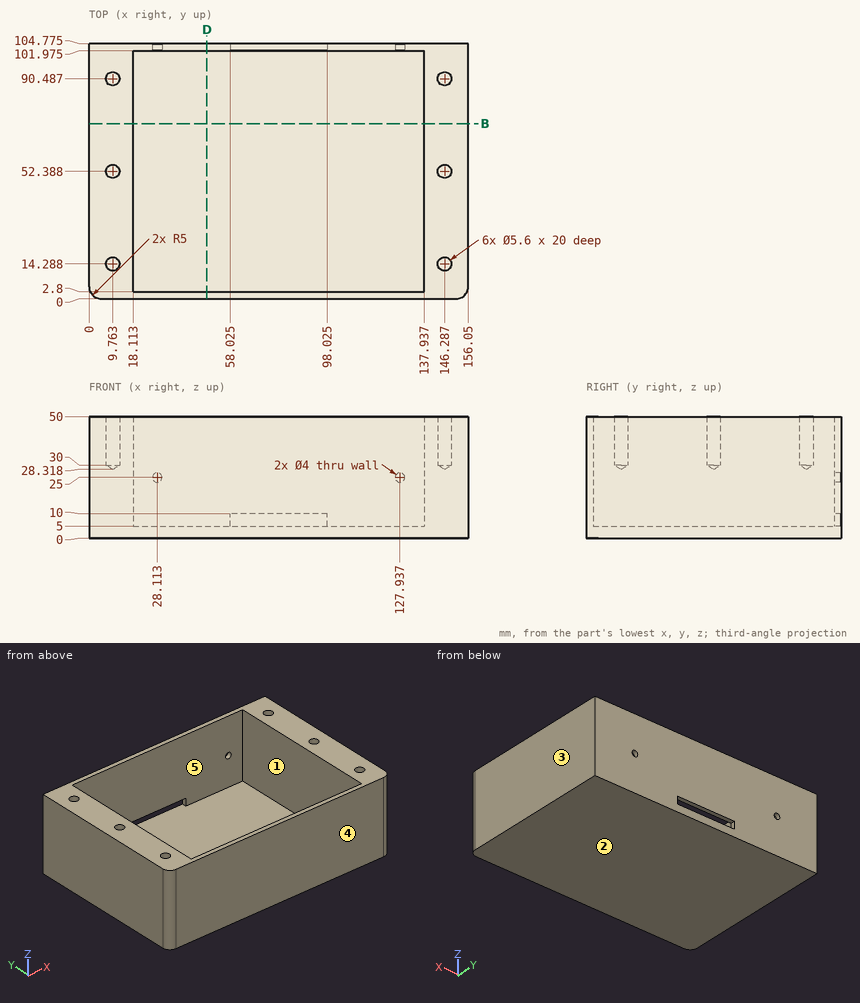
Study the drawing (mm; zero at the part's minimum x, y, z) and answer. A direction names the side the tool comes from. Give positions to 0.01 mm unless a question says otherwise; leave off trailing zeros. Write each loop counter-clockwise with the first axis right and the second up, starting at its lowest first coordinate (ties: lowest second). Pieces come first, ordered by that corner, then holes. Notation, with made-up numbers: (-0.75, -12.5) -> (40.25, -12.5) arc R27 cw to (40.25, 5.5) -> close; hole circle Ø9 at (24, 23.5). An arc over 180 degrees is marked (long way). Answer as a JSON object with one key per item and string values. Group by question number.
1) A tool of negligible diameter and unlimited length cuts with its end or side. For the marked faces 4 and 5, from which of +Z, -Z, +X, -X, +Y, -Y can it reach the whole face along a straight path? Write none if from no direction.
2) The mould has two halves that part along X. Classify the marked faces 1, 2 and 3: +X half, -X half, draft (parallel to the pull), parting line (faces both ways), or undercut.
3) Find section D-D (x = 48.5). Write down the section's boundary in (y, z) (1 decimal), and give its area (3 significant figures).
4) Each of these flat-tipped pins is pushed along its axis until it touches: P1, Ø10, axis at x = 90.5, y = 29.5, coming from the +Z side; P2, Ø5, axis at x = 9.763, y = 52.388, coming from the +Z side. Where does it stop, or does it pass through?
5) Consider L1, parallel to X at y = 46.5, z = 36.5; L2, parallel to Y at x = 110, z = 26.5 (1 decimal); L3, parallel to Z at x = 100.5, y = 76. Determine where each line is inside the solid, lowest interval first. Write a range as from..to.
6) Find section B-B (y = 72). Write down the section's boundary in (x, z), and give its area (3 significant figures).
Values follow:
{
 "1": {"face 4": "+Z, -Z, +X, -X, -Y", "face 5": "+Z"},
 "2": {"face 1": "undercut", "face 2": "draft", "face 3": "+X half"},
 "3": {"outline": "(0, 0) -> (104.8, 0) -> (104.8, 50) -> (102, 50) -> (102, 5) -> (2.8, 5) -> (2.8, 50) -> (0, 50) -> close", "area": "776 mm2"},
 "4": {"P1": "stops at z = 5", "P2": "stops at z = 29.82"},
 "5": {"L1": "x = 0..18.11, 137.94..156.05", "L2": "y = 0..2.8, 102..104.8", "L3": "z = 0..5"},
 "6": {"outline": "(0, 0) -> (156.05, 0) -> (156.05, 50) -> (137.94, 50) -> (137.94, 5) -> (18.11, 5) -> (18.11, 50) -> (0, 50) -> close", "area": "2,410 mm2"}
}
